from build123d import *

# Parameters (mm, degrees)
F0_W     = 76.2
F0_H     = 76.2
F0_R     = 12.7
F1_DEPTH = 25.4


with BuildPart() as f1:
    # F0 (on Front) → F1 (new body)
    with BuildSketch(Plane.XZ):
        Rectangle(F0_W, F0_H)
        Circle(F0_R, mode=Mode.SUBTRACT)
    extrude(amount=-F1_DEPTH)


solid = f1.part
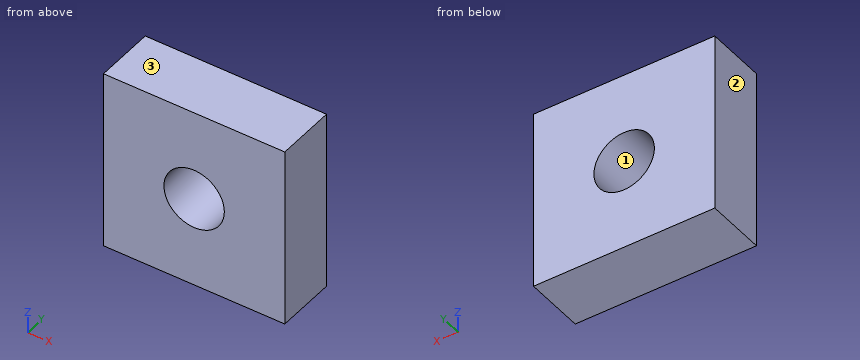
Part model, mm, in its own coordinate system. Face numbers are marked on the shaded views. Round coordinates to 2 decimals unless told otherwise and drop trailing zeros. Write each loop counter-clockwise with the first axis right and the second up, starting at its lowest first coordinate (ties: lowest second). Pieces come first, ordered by that corner, then holes. Notation, with made-up numbers: M -12,58.25 L 13,58.25 A15 cw 13,66.25 Z; hole C 52.5,-9 d10. An arc over 180 degrees is marked long. Return JSON: item names as keys, results as strings. Group by question number.
(1) Saw through at A-A on x = 0. Write the cut outline in (y, z).
(2) Drill centre lines: probe 1 along Z at (x, y) = (0, 18.25); probe 2 along Z at (x, y) = (-10.5, 17.5). Where is each one in solid material? Low to high.
(3) Pin check, flat tip, straight feed: pin 1 Ø12 at (x, z) = (-5, -2) entering from -Y. Stop position of the tip, or through.
(4) Saw through at B-B on z = 0. Write the cut outline in (x, y), then the cut area to 3 significant figures.
(5) Saw through at C-C on y = 3. Write the cut outline in (x, z), then the cut area to 3 significant figures.
(6) Two-plate mould, pull along X, no slides. Class the marked faces 1, 2 and 3: +X half, -X half, draft (parallel to the pull), parting line (faces both ways), or undercut.
Returned:
{
 "1": {"outline": "M 0,-38.1 L 25.4,-38.1 L 25.4,-12.7 L 0,-12.7 Z; M 0,12.7 L 25.4,12.7 L 25.4,38.1 L 0,38.1 Z"},
 "2": {"probe 1": "-38.1 to -12.7, 12.7 to 38.1", "probe 2": "-38.1 to -7.14, 7.14 to 38.1"},
 "3": {"pin 1": "through"},
 "4": {"outline": "M -38.1,0 L -12.7,0 L -12.7,25.4 L -38.1,25.4 Z; M 12.7,0 L 38.1,0 L 38.1,25.4 L 12.7,25.4 Z", "area": "1,290 mm²"},
 "5": {"outline": "M -38.1,-38.1 L 38.1,-38.1 L 38.1,38.1 L -38.1,38.1 Z; hole C 0,0 d25.4", "area": "5,300 mm²"},
 "6": {"face 1": "undercut", "face 2": "-X half", "face 3": "draft"}
}
